Check sheet for the modelled part. Datum: model origin and axes. Units: mm. A direction names the side the tool comes from. Round coordinates to 2 decimals unless told otherwise and drop trailing zeros. Loops run counter-clockwise (first coordinate to the right, second up) from the corner with the lowest first, then second, coordinate; pieces in that order, holes last. Notation, with made-up numbers: (28.5, -2) - (39.5, -2) arc R18 ccw to (39.5, 17) - close; hole circle Ø3 at (13, -20.75). An arc over 180 degrees is marked (long way). Answer in a Markdown table with one row per item. Add a question column.
(1) Mould release check, pull along X, two halves, no side actions. Record for faces 1 (the flat face through (0, -36, -2.595)), 2 (the flat face through (-21, 36, 27)), 3 (the flat face through (32, 0, 0)), 4 (the cylindrical face through (33.38, -33.73, 1.27)): +X half, -X half, draft (parallel to the pull), parting line (faces both ways), or undercut.
(2) Gauge pin test, flat ends, axial feed: pin 1 (4 mm diameter, centred on x = 15.205, z = 35, fed in from -Y); pin 2 (12 mm diameter, centred on x = -28.5, y = -22, fed in from +Z); pin 3 (4 mm diameter, centred on y = 34, z = 26.5, fed in from +X); pin 4 (2 mm diameter, centred on y = 29.5, z = 6, fed in from +X). Record the tip position at first contact, or that the pin passes through.
(3) Thickness scan on line 1 along X through (y, z) = (-37.5, 35); line 2 along Y through (x, z) = (5.5, 20.5); line 3 along Z through (x, y) = (0, -34) (3 decimals). Record the ranges inside material, lowest first.
(4) Cross-section at A-A on y = 14. Enter the section's corners in (x, z).
(5) Cross-section at B-B on z = 0. Enter the section's corners in (x, y) (3 decimals).
(6) Cross-section at D-D on z = 13. Enter the section's corners in (x, y).
(7) Cross-section at C-C on x = 0. Enter the section's corners in (y, z) (3 decimals), then the cut area to 3 significant figures.
(8) Access from +Z, -Z, +X, -X, +Y, -Y to the whole of each face (thin tool, end or side, straight path). Record for faces 5 (the flat face through (21, -36, 27)), 6 (the flat face through (-21, -36, 27)), 7 (the flat face through (0, 32, 15)).
from build123d import *

# Parameters (mm, degrees)
ESQUISSE1_W                             = 80
ESQUISSE1_H                             = 80
ESQUISSE1_W_2                           = 64
ESQUISSE1_H_2                           = 64
BOSS_EXTRU_1_DEPTH                      = 15
ESQUISSE7_W                             = 42
ESQUISSE7_H                             = 8
BOSS_EXTRU_4_DEPTH                      = 30
PER_AGE_POUR_CROUS_AUTO_BLOQUANTS_300_D = 4.7625
CONG_1_R                                = 10
CONG_1_OF_SYM_TRIE2_R                   = 10
CONG_2_R                                = 22
CONG_3_R                                = 14
CONG_4_R                                = 5
ENL_V_MAT_EXTRU_3_DEPTH                 = 124.389626959


with BuildPart() as part:
    # Esquisse1 → Boss.-Extru.1 (new, symmetric)
    with BuildSketch(Plane.XY):
        Rectangle(ESQUISSE1_W, ESQUISSE1_H)
        Rectangle(ESQUISSE1_W_2, ESQUISSE1_H_2, mode=Mode.SUBTRACT)
    extrude(amount=BOSS_EXTRU_1_DEPTH, both=True)

    # Esquisse7 → Boss.-Extru.4 (add)
    with BuildSketch(Plane.XY.offset(15)):
        with Locations((0, 36)):
            Rectangle(ESQUISSE7_W, ESQUISSE7_H)
    boss_extru_4 = extrude(amount=BOSS_EXTRU_4_DEPTH)

    # Perçage pour écrous auto-bloquants 300® #6 (SP)1 (through all)
    with Locations(Plane(origin=(0, 40, 0), x_dir=(0, 0, -1), z_dir=(0, 1, 0))):
        with Locations((-35, -15.205), (-35, 15.205)):
            per_age_pour_crous_auto_bloquants_300 = Hole(PER_AGE_POUR_CROUS_AUTO_BLOQUANTS_300_D / 2)

    # Congé1
    cong_1_edges = [part.edges().sort_by_distance(p)[0] for p in [
        (21, 36, 45),
        (-21, 36, 45),
    ]]
    fillet(cong_1_edges, radius=CONG_1_R)

    # Symétrie2: Boss.-Extru.4, Perçage pour écrous auto-bloquants 300® #6 (SP)1 across plane
    add(boss_extru_4.mirror(Plane.ZX))
    add(per_age_pour_crous_auto_bloquants_300.mirror(Plane.ZX), mode=Mode.SUBTRACT)

    # Congé1 of Symétrie2
    cong_1_of_sym_trie2_edges = [part.edges().sort_by_distance(p)[0] for p in [
        (21, -36, 45),
        (-21, -36, 45),
    ]]
    fillet(cong_1_of_sym_trie2_edges, radius=CONG_1_OF_SYM_TRIE2_R)

    # Congé2
    cong_2_edges = [part.edges().sort_by_distance(p)[0] for p in [
        (40, -40, 0),
        (-40, -40, 0),
        (-40, 40, 0),
        (40, 40, 0),
    ]]
    fillet(cong_2_edges, radius=CONG_2_R)

    # Congé3
    cong_3_edges = [part.edges().sort_by_distance(p)[0] for p in [
        (-32, 32, 0),
        (-32, -32, 0),
        (32, -32, 0),
        (32, 32, 0),
    ]]
    fillet(cong_3_edges, radius=CONG_3_R)

    # Congé4
    cong_4_edges = [part.edges().sort_by_distance(p)[0] for p in [
        (-21, -35.734644524, 15),
        (-21, 35.734644524, 15),
        (21, 35.734644524, 15),
        (21, -35.734644524, 15),
    ]]
    fillet(cong_4_edges, radius=CONG_4_R)

    # Esquisse11 → Enlèv. mat.-Extru.3 (cut, through all)
    with BuildSketch(Plane(origin=(0, -40, -40), x_dir=(1, 0, 0), z_dir=(0, 1, 0))):
        with BuildLine():
            Line((1.964942747, -37.405), (-1.964942747, -37.405))
            ThreePointArc((-1.964942747, -37.405), (0, -43.255), (1.964942747, -37.405))
        make_face()
    extrude(amount=ENL_V_MAT_EXTRU_3_DEPTH, mode=Mode.SUBTRACT)


solid = part.part
Answers:
| question | item | result |
|---|---|---|
| 1 | face 1 | undercut |
| 1 | face 2 | -X half |
| 1 | face 3 | undercut |
| 1 | face 4 | +X half |
| 2 | pin 1 | passes through |
| 2 | pin 2 | stops at z = 15 |
| 2 | pin 3 | stops at x = 21 |
| 2 | pin 4 | stops at x = 37.33 |
| 3 | line 1 | x = -21 to -17.59, -12.82 to 12.82, 17.59 to 21 |
| 3 | line 2 | y = -40 to -32, 32 to 40 |
| 3 | line 3 | z = -15 to -2.595, 3.255 to 45 |
| 4 | outline | (-40, -15) - (-32, -15) - (-32, 15) - (-40, 15) - close; (32, -15) - (40, -15) - (40, 15) - (32, 15) - close |
| 5 | outline | (-40, -18) arc R22 ccw to (-18, -40) - (-3.255, -40) - (-3.255, -32) - (-18, -32) arc R14 cw to (-32, -18) - (-32, 18) arc R14 cw to (-18, 32) - (-3.255, 32) - (-3.255, 40) - (-18, 40) arc R22 ccw to (-40, 18) - close; (3.255, -40) - (18, -40) arc R22 ccw to (40, -18) - (40, 18) arc R22 ccw to (18, 40) - (3.255, 40) - (3.255, 32) - (18, 32) arc R14 cw to (32, 18) - (32, -18) arc R14 cw to (18, -32) - (3.255, -32) - close |
| 6 | outline | (-40, -18) arc R22 ccw to (-18, -40) - (18, -40) arc R22 ccw to (40, -18) - (40, 18) arc R22 ccw to (18, 40) - (-18, 40) arc R22 ccw to (-40, 18) - close; hole (-32, -18) arc R14 ccw to (-18, -32) - (18, -32) arc R14 ccw to (32, -18) - (32, 18) arc R14 ccw to (18, 32) - (-18, 32) arc R14 ccw to (-32, 18) - close |
| 7 | outline | (-40, -15) - (-32, -15) - (-32, -2.595) - (-40, -2.595) - close; (-40, 3.255) - (-32, 3.255) - (-32, 45) - (-40, 45) - close; (32, -15) - (40, -15) - (40, -2.595) - (32, -2.595) - close; (32, 3.255) - (40, 3.255) - (40, 45) - (32, 45) - close |
| 7 | area | 866 mm^2 |
| 8 | face 5 | +Z, +X, +Y, -Y |
| 8 | face 6 | +Z, -X, +Y, -Y |
| 8 | face 7 | +Z, -Z |
